Geometry check sheet. Reference: drawing and pictorial views, mm from the part's lowest x, y, z. A direction names the side the tool comes from. Give positions to 0.01 mm unless a question says otherwise; leave off trailing zeros. Loops run counter-clockwise (first coordinate to the right, second up) from the corner with the lowest first, then second, coordinate; pieces in that order, holes last. Notation, with made-up numbers: (65.5, 7.25) - (117.5, 7.25) arc R14 ccw to (117.5, 20.25) - close; hole circle Ø11 at (59, 12.25). An arc over 180 degrees is marked (long way). Put each result on its own line as item: value. Start each with the question number.
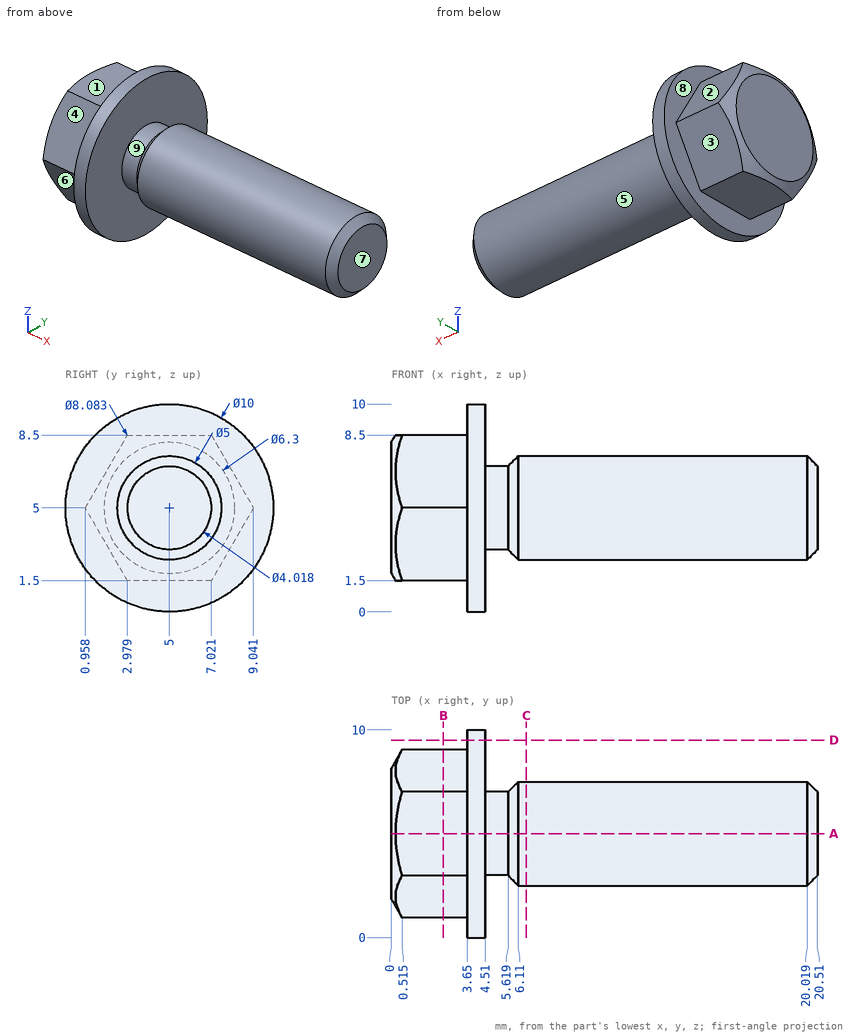
1) Section check D-D, the plane y = 9.5. Enter the section's corners in (x, z).
2) Section check B-B, the plane x = 2.5. Enter the section's corners in (y, z).
3) Depth check by flat-ended pin: P1, Ø1, axis at y = 1.5, z = 6, coming from the +X side; P2, Ø2, axis at x = 2.5, y = 1.5, coming from the +Z side; P3, Ø1.7, axis at x = 2.5, y = 4.5, coming from the -Z side. Enter the tip coordinate at first touch or a pass-through.
4) Scan lines: line 1 along X through (y, z) = (8, 2.75); line 2 along Y through (x, z) = (19.25, 5); line 3 along Z through (x, y) = (2.5, 5.75). Record each from-to range of solid material in increasing order. Write a range as from..to.
5) Set-up check for the marked faces 1, 2, 3, 4 and 5: record each of +Z, -Z, +X, -X, +Y, -Y from which the full face is reachable in a straight line by a thin tool's end or side.
6) Draft check along X on the marked faces 6, 7, 8 and 9. Enter one of: pulls with the +X half, pulls with the -X half, needs draft (parallel to the pull), parting line crosses it, or undercut.
7) Section check A-A, the plane y = 5. Enter the section's corners in (x, z).
8) Section check C-C, the plane x = 6.5. Enter the section's corners in (y, z).
Results are:
1. outline: (3.65, 2.82) - (4.51, 2.82) - (4.51, 7.18) - (3.65, 7.18) - close
2. outline: (0.96, 5) - (2.98, 1.5) - (7.02, 1.5) - (9.04, 5) - (7.02, 8.5) - (2.98, 8.5) - close
3. P1: stops at x = 4.51
3. P2: stops at z = 7.67
3. P3: stops at z = 1.5
4. line 1: x = 3.65..4.51
4. line 2: y = 2.5..7.5
4. line 3: z = 1.5..8.5
5. face 1: +Z, -X, +Y, -Y
5. face 2: +Z, -X, +Y
5. face 3: -Z, -X, +Y
5. face 4: +Z, -X, -Y
5. face 5: +X
6. face 6: needs draft
6. face 7: pulls with the +X half
6. face 8: pulls with the -X half
6. face 9: undercut
7. outline: (0, 1.85) - (0.2, 1.5) - (3.65, 1.5) - (3.65, 0) - (4.51, 0) - (4.51, 2.99) - (5.62, 2.99) - (6.11, 2.5) - (20.02, 2.5) - (20.51, 2.99) - (20.51, 7.01) - (20.02, 7.5) - (6.11, 7.5) - (5.62, 7.01) - (4.51, 7.01) - (4.51, 10) - (3.65, 10) - (3.65, 8.5) - (0.2, 8.5) - (0, 8.15) - close
8. outline: circle Ø5 at (5, 5)
